The listing builds one solid part. Answer for the finished solid, in the listing's coordinates (mm). Face numbers are marked on the shaded views. A direction names the side the tool comes from. Round coordinates to 2 decimals unless told otherwise and drop trailing zeros. Loops run counter-clockwise (first coordinate to the right, second up) from the corner with the lowest first, then second, coordinate; pieces in that order, holes last. Notation, with made-up numbers: M 75,83 L 102,83 A30 ccw 102,112 Z; hole C -34,74.5 d3. An arc over 180 degrees is marked long. Answer as a JSON object with one key per item and string values.
```python
from build123d import *

# Parameters (mm, degrees)
F0_R     = 35
F0_R_2   = 25.35
F1_DEPTH = 11.75
F0_R_3   = 3.8
F2_DEPTH = 25
F3_R     = 2


with BuildPart() as f1:
    # F0 (on Top) → F1 (new body)
    with BuildSketch(Plane.XY):
        Circle(F0_R)
        Circle(F0_R_2, mode=Mode.SUBTRACT)
    extrude(amount=F1_DEPTH)

    # F0 (on Top) → F2 (join)
    with BuildSketch(Plane.XY):
        Circle(F0_R_2)
        Circle(F0_R_3, mode=Mode.SUBTRACT)
    extrude(amount=F2_DEPTH)

    # F3
    f3_edges = [f1.edges().sort_by_distance(p)[0] for p in [
        (-35, 0, 11.75),
        (-25.35, 0, 25),
        (-3.8, 0, 25),
    ]]
    fillet(f3_edges, radius=F3_R)


solid = f1.part
```
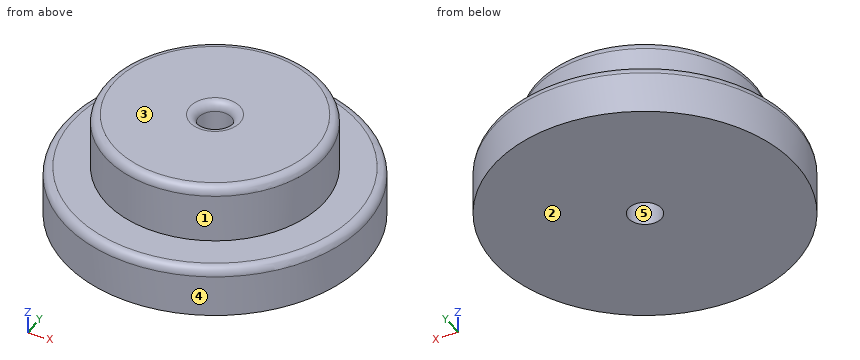
Item 1: Which of the six approach directions +Z, -Z, +X, -X, +Y, -Y give full straight-line access (tool end or side, diameter ignored) to the marked faces 1 and 2?
Values follow:
{"face 1": "+Z", "face 2": "-Z, +X, -X, +Y, -Y"}
Item 2: Flat-ended cylindrical pins translate along their axes: P1, Ø10, axis at y = -10.5, z = 12.5, coming from the +X side; P2, Ø3, axis at y = -8, z = 20, coming from the +X side; P3, Ø2, axis at y = 7, z = 8.5, coming from the +X side; P4, Ø6, axis at x = 0, y = 0, coming from the -Z side. Find the tip coordinate at first contact, or state that the pin passes through.
Values follow:
{"P1": "x = 34.44", "P2": "x = 24.5", "P3": "x = 34.48", "P4": "through"}
Item 3: Straight lines are drawn through the part: line 1 (Y direction, x = 0, z = 4.75); line 2 (Y direction, x = 0, z = 16); line 3 (Z direction, x = 22.5, y = 24.5). For each, find the intervals that lie inside material, in ascending order.
Values follow:
{"line 1": "-35 to -3.8, 3.8 to 35", "line 2": "-25.35 to -3.8, 3.8 to 25.35", "line 3": "0 to 11.73"}
Item 4: The part is cut by section A-A (y = 0). Give the vertices of the cut face in (x, z), then the cut area to 3 significant figures.
Values follow:
{"outline": "M -35,0 L -3.8,0 L -3.8,23 A2 ccw -5.8,25 L -23.35,25 A2 ccw -25.35,23 L -25.35,11.75 L -33,11.75 A2 ccw -35,9.75 Z; M 3.8,0 L 35,0 L 35,9.75 A2 ccw 33,11.75 L 25.35,11.75 L 25.35,23 A2 ccw 23.35,25 L 5.8,25 A2 ccw 3.8,23 Z", "area": "1,300 mm^2"}
Item 5: The part is cut by section C-C (z = 17). Give the vertices of the cut face in (x, y).
Values follow:
{"outline": "C 0,0 d50.7; hole C 0,0 d7.6"}
Item 6: Determine the mould class of the marked faces 3, 4 and 5 for opening direction X: released by +X, released by -X, zero draft, split by the parting line, or undercut.
Values follow:
{"face 3": "zero draft", "face 4": "split by the parting line", "face 5": "undercut"}
